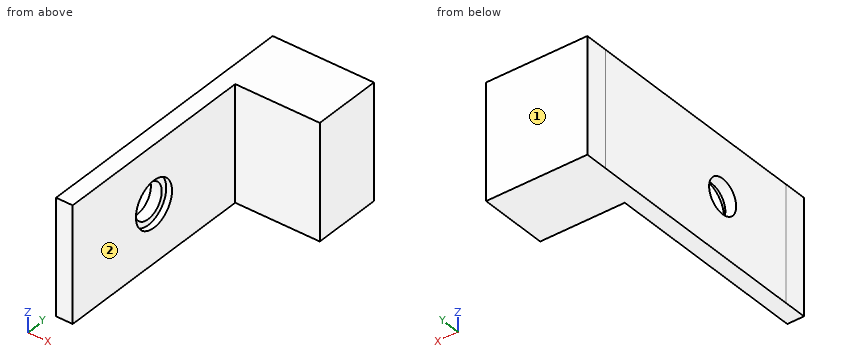
from build123d import *

# Parameters (mm, degrees)
ESQUISSE1_W             = 30
ESQUISSE1_H             = 24
BOSS_EXTRU_1_DEPTH      = 10
ESQUISSE2_W             = 20
ESQUISSE2_H             = 20
ENL_V_MAT_EXTRU_1_DEPTH = 10
ESQUISSE3_W             = 7.346397708
ESQUISSE3_H             = 18
ENL_V_MAT_EXTRU_2_DEPTH = 10
ESQUISSE5_W             = 21.205400457
ESQUISSE5_H             = 24
ENL_V_MAT_EXTRU_3_DEPTH = 10
ESQUISSE6_R             = 2
ENL_V_MAT_EXTRU_4_DEPTH = 0.5
ESQUISSE7_R             = 1.5
ENL_V_MAT_EXTRU_5_DEPTH = 10.5


with BuildPart() as part:
    # Esquisse1 → Boss.-Extru.1 (new body)
    with BuildSketch(Plane.XY):
        with Locations((3.298240101, -8.976744186)):
            Rectangle(ESQUISSE1_W, ESQUISSE1_H)
    extrude(amount=BOSS_EXTRU_1_DEPTH)

    # Esquisse2 → Enlèv. mat.-Extru.1 (cut)
    with BuildSketch(Plane.XY.offset(10)):
        with Locations((-0.490787108, -8.976744186)):
            Rectangle(ESQUISSE2_W, ESQUISSE2_H)
    extrude(amount=-ENL_V_MAT_EXTRU_1_DEPTH, mode=Mode.SUBTRACT)

    # Esquisse3 → Enlèv. mat.-Extru.2 (cut)
    with BuildSketch(Plane.XY.offset(10)):
        with Locations((14.625041247, -11.976744186)):
            Rectangle(ESQUISSE3_W, ESQUISSE3_H)
    extrude(amount=-ENL_V_MAT_EXTRU_2_DEPTH, mode=Mode.SUBTRACT)

    # Esquisse5 → Enlèv. mat.-Extru.3 (cut)
    with BuildSketch(Plane.XY.offset(10)):
        with Locations((-1.09905967, -8.976744186)):
            Rectangle(ESQUISSE5_W, ESQUISSE5_H)
    extrude(amount=-ENL_V_MAT_EXTRU_3_DEPTH, mode=Mode.SUBTRACT)

    # Esquisse6 → Enlèv. mat.-Extru.4 (cut)
    with BuildSketch(Plane(origin=(10.951842393, 0, 0), x_dir=(0, 0, -1), z_dir=(1, 0, 0))):
        with Locations((-5, -11.976744186)):
            Circle(ESQUISSE6_R)
    extrude(amount=-ENL_V_MAT_EXTRU_4_DEPTH, mode=Mode.SUBTRACT)

    # Esquisse7 → Enlèv. mat.-Extru.5 (cut)
    with BuildSketch(Plane(origin=(10.451842393, 0, 0), x_dir=(0, 0, -1), z_dir=(1, 0, 0))):
        with Locations((-5, -11.976744186)):
            Circle(ESQUISSE7_R)
    extrude(amount=-ENL_V_MAT_EXTRU_5_DEPTH, mode=Mode.SUBTRACT)


solid = part.part
CAD build for the part. Positions are in the model's coordinates, mm. Face numbers are marked on the shaded views. A direction names the side the tool comes from. Round coordinates to 2 decimals unless told otherwise and drop trailing zeros. Write each loop counter-clockwise with the first axis right and the second up, starting at its lowest first coordinate (ties: lowest second). Pieces come first, ordered by that corner, then holes.
(1) Slice it at C-C, the plane y = -8.75. Write the cut outline in (x, z).
(2) Probe line 1 along Y through (x, z) = (10.75, 5); line 2 along Y through (x, z) = (9.8, 5); line 3 along X through (y, z) = (-18.5, 2). List the from-to ranges inside material, lowest first.
(3) 3-axis set-ups, long thin cutter, end or side, ignore diameter. For the marked faces 1 and 2: which of +Z, -Z, +X, -X, +Y, -Y reach the whole face in a straight line?
(4) Slice it at D-D, the plane x = 15.5. Write the cut outline in (y, z).
(5) Drop flat-ended pins along their axis: P1, Ø5, axis at y = -13, z = 3.5, coming from the +X side; P2, Ø5, axis at y = -6.5, z = 6, coming from the -X side; P3, Ø3.5, axis at x = 15, z = 7, coming from the -Y side. Give the stop position or say it passes through.
From the geometry:
1. outline: (9.51, 0) - (10.95, 0) - (10.95, 10) - (9.51, 10) - close
2. line 1: y = -20.98 to -13.98, -9.98 to 3.02
2. line 2: y = -20.98 to -13.48, -10.48 to 3.02
2. line 3: x = 9.51 to 10.95
3. face 1: +Z, -Z, +X, -X, +Y
3. face 2: +Z, -Z, +X, -Y
4. outline: (-2.98, 0) - (3.02, 0) - (3.02, 10) - (-2.98, 10) - close
5. P1: stops at x = 10.95
5. P2: stops at x = 9.51
5. P3: stops at y = -2.98
